Build history of the part. All positions in model axes, mm. Face numbers are marked on the shaded views. A direction names the side the tool comes from. Round coordinates to 2 decimals unless told otherwise and drop trailing zeros. Write each loop counter-clockwise with the first axis right and the second up, starting at its lowest first coordinate (ties: lowest second). Pieces come first, ordered by that corner, then holes. Notation, with made-up numbers: (88, 40) - (136, 40) arc R30 ccw to (136, 75) - close; hole circle Ø11 at (70.5, -2). An arc over 180 degrees is marked (long way). One line per question, with ' | ' between items.
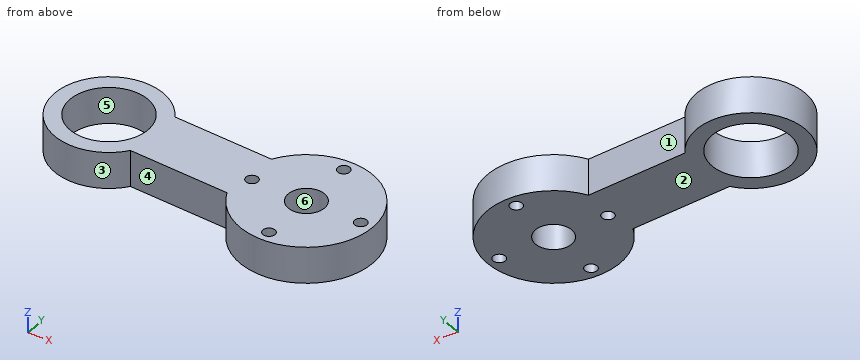
from build123d import *

# Parameters (mm, degrees)
BOSS_EXTRU_1_DEPTH      = 6
ESQUISSE2_R             = 1.005
ESQUISSE2_R_2           = 3
ENL_V_MAT_EXTRU_1_DEPTH = 6
ESQUISSE3_R             = 9
BOSS_EXTRU_2_DEPTH      = 6
ESQUISSE5_R             = 6.45
ENL_V_MAT_EXTRU_2_DEPTH = 6


with BuildPart() as part:
    # Esquisse1 → Boss.-Extru.1 (new body)
    with BuildSketch(Plane.XY):
        with BuildLine():
            Line((-10.02588737, -4.525658234), (-40.02588737, -3.070914704))
            Line((-40.02588737, -3.070914704), (-39.541047229, 6.929085296))
            Line((-39.541047229, 6.929085296), (-9.541047229, 5.474341766))
            ThreePointArc((-9.541047229, 5.474341766), (10.987093901, -0.532698415), (-10.02588737, -4.525658234))
        make_face()
    extrude(amount=BOSS_EXTRU_1_DEPTH)

    # Esquisse2 → Enlèv. mat.-Extru.1 (cut)
    with BuildSketch(Plane.XY.offset(6)):
        with Locations((0, 9)):
            Circle(ESQUISSE2_R)
        with Locations((9, 0)):
            Circle(ESQUISSE2_R)
        with Locations((0, -9)):
            Circle(ESQUISSE2_R)
        with Locations((-9, 0)):
            Circle(ESQUISSE2_R)
        with Locations((-33.790793572, 1.632611651)):
            Circle(ESQUISSE2_R)
        Circle(ESQUISSE2_R_2)
    extrude(amount=-ENL_V_MAT_EXTRU_1_DEPTH, mode=Mode.SUBTRACT)

    # Esquisse3 → Boss.-Extru.2 (add)
    with BuildSketch(Plane(origin=(0, 0, 0), x_dir=(-1, 0, 0), z_dir=(0, 0, -1))):
        with Locations((33.790793572, 1.632611651)):
            Circle(ESQUISSE3_R)
    extrude(amount=-BOSS_EXTRU_2_DEPTH)

    # Esquisse5 → Enlèv. mat.-Extru.2 (cut)
    with BuildSketch(Plane(origin=(0, 0, 0), x_dir=(-1, 0, 0), z_dir=(0, 0, -1))):
        with Locations((33.790793572, 1.632611651)):
            Circle(ESQUISSE5_R)
    extrude(amount=-ENL_V_MAT_EXTRU_2_DEPTH, mode=Mode.SUBTRACT)


solid = part.part
Q1. Which spindle directions (+Z, -Z, +X, -X, +Y, -Y) get a long thin tool onto all of the face, cutting with end or side? Do the marked faces 1 and 2. Say none if no direction does.
Found:
face 1: +Z, -Z, +Y | face 2: -Z, +X, -X, +Y, -Y
Q2. Saw through at C-C, the plane y = 9. List the corners of the cut face in (x, z) (1 decimal), then the cut area to 3 significant figures.
Found:
outline: (-39, 0) - (-28.6, 0) - (-28.6, 6) - (-39, 6) - close; (-6.3, 0) - (-1, 0) - (-1, 6) - (-6.3, 6) - close; (1, 0) - (6.3, 0) - (6.3, 6) - (1, 6) - close | area: 126 mm^2
Q3. Drill centre lines: L1, parallel to Y at x = 0, z = 1.6 (3 decimals); L2, parallel to X at y = 2, z = 2.3; L3, parallel to X at y = 2.5, z = 4.3. Where is each one in solid material? Low to high. Write a range as from..to.
Found:
L1: -11..-10.005, -7.995..-3, 3..7.995, 10.005..11 | L2: -42.78..-40.23, -27.35..-2.24, 2.24..10.82 | L3: -42.75..-40.18, -27.4..-1.66, 1.66..10.71
Q4. Drop flat-ended pins along their axis: pin 1 (12 mm diameter, centred on x = -1, y = -5.5, fed in from -Z); pin 2 (3 mm diameter, centred on y = 6.5, z = 2, fed in from +X); pin 3 (1.5 mm diameter, centred on x = -8, z = 4, fed in from +Y). Give the stop position or say it passes through.
Found:
pin 1: z = 0 | pin 2: x = 9.8 | pin 3: y = 8.27
Q5. Pull direction Y, two halves, no side cores. Call the marked faces 3, 4, 5 and 6: +Y half, -Y half, draft (parallel to the pull), parting line (faces both ways), or undercut.
Found:
face 3: parting line | face 4: -Y half | face 5: undercut | face 6: undercut
Q6. Saw through at A-A, the plane x = -35.5. List the corners of the cut face in (y, z).
Found:
outline: (-7.2, 0) - (-4.59, 0) - (-4.59, 6) - (-7.2, 6) - close; (7.85, 0) - (10.47, 0) - (10.47, 6) - (7.85, 6) - close
Q7. Saw through at D-D, the plane x = 0. List the corners of the cut face in (y, z) (3 decimals), then the cut area to 3 significant figures.
Found:
outline: (-11, 0) - (-10.005, 0) - (-10.005, 6) - (-11, 6) - close; (-7.995, 0) - (-3, 0) - (-3, 6) - (-7.995, 6) - close; (3, 0) - (7.995, 0) - (7.995, 6) - (3, 6) - close; (10.005, 0) - (11, 0) - (11, 6) - (10.005, 6) - close | area: 71.9 mm^2
Q8. Saw through at B-B, the plane y = -8.5. List the corners of the cut face in (x, z), then the cut area to 3 significant figures.
Found:
outline: (-6.98, 0) - (-0.87, 0) - (-0.87, 6) - (-6.98, 6) - close; (0.87, 0) - (6.98, 0) - (6.98, 6) - (0.87, 6) - close | area: 73.3 mm^2
